Here's the drawing with two shaded views (mm, measured from the low corner). I have some questions. Round coordinates to 2 decimals unless told otherwise and drop trailing zeros. Loops run counter-clockwise (first coordinate to the right, second up) from the corner with the lowest first, then second, coordinate; pieces in that order, holes last. Notation, with made-up numbers: (40, -11.75) -> (83, -11.75) arc R35 cw to (83, 26.25) -> close; hole circle Ø5 at (39.25, 76). An arc over 180 degrees is marked (long way). Use a Markdown table: item, result.
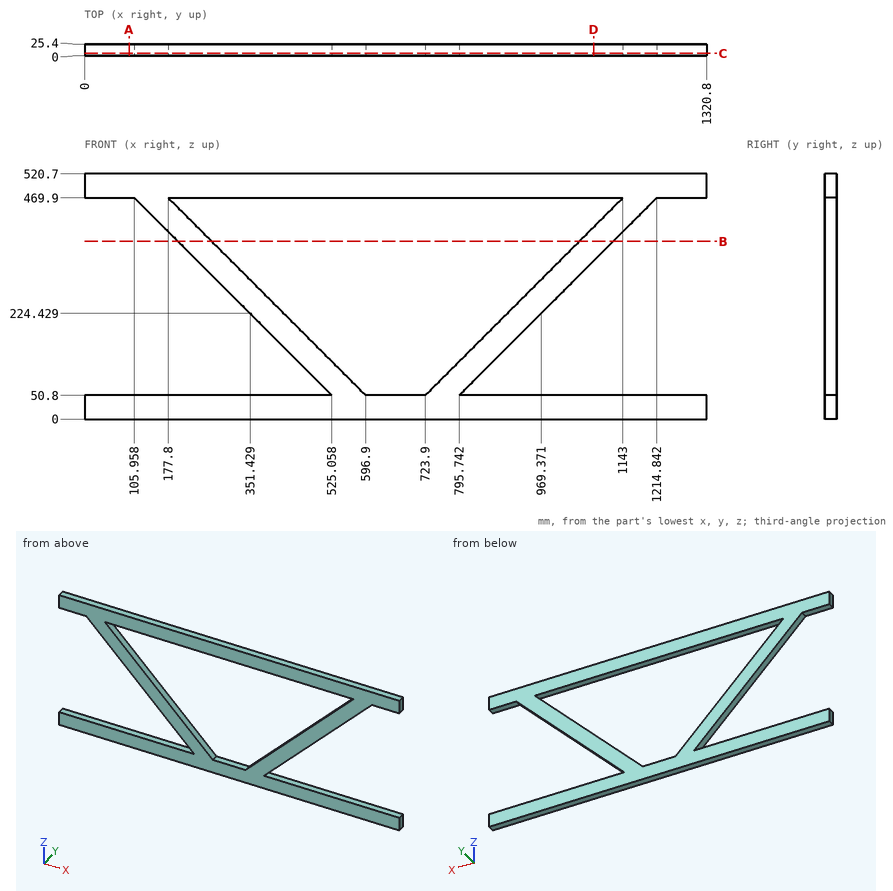
1. I want a section at B-B (z = 377.5). Please give me the cut outline in (x, y).
Answer sheet:
| item | result |
|---|---|
| outline | (198.36, 0) -> (270.2, 0) -> (270.2, 25.4) -> (198.36, 25.4) -> close; (1050.6, 0) -> (1122.44, 0) -> (1122.44, 25.4) -> (1050.6, 25.4) -> close |
2. I want a section at A-A (x = 94.5). Please give me the cut outline in (y, z), plus the area to 3 significant figures.
Answer sheet:
| item | result |
|---|---|
| outline | (0, 0) -> (25.4, 0) -> (25.4, 50.8) -> (0, 50.8) -> close; (0, 469.9) -> (25.4, 469.9) -> (25.4, 520.7) -> (0, 520.7) -> close |
| area | 2,580 mm² |
3. I want a section at D-D (x = 1081). Please give me the cut outline in (y, z), plus the area to 3 significant figures.
Answer sheet:
| item | result |
|---|---|
| outline | (0, 0) -> (25.4, 0) -> (25.4, 50.8) -> (0, 50.8) -> close; (0, 336.06) -> (25.4, 336.06) -> (25.4, 407.9) -> (0, 407.9) -> close; (0, 469.9) -> (25.4, 469.9) -> (25.4, 520.7) -> (0, 520.7) -> close |
| area | 4,410 mm² |
4. I need wall thicknesses on line 1 (Z direction, x = 486, y = 9); line 2 (Z direction, x = 1037, y = 14.75); line 3 (Z direction, x = 636, y = 6.75). Which ranges of each line are inside material? Lowest first, please.
Answer sheet:
| item | result |
|---|---|
| line 1 | z = 0 to 50.8, 89.86 to 161.7, 469.9 to 520.7 |
| line 2 | z = 0 to 50.8, 292.06 to 363.9, 469.9 to 520.7 |
| line 3 | z = 0 to 50.8, 469.9 to 520.7 |
5. Will these pins go through, and if not, where does the flat tip stop? pin 1 Ø5 at (y, z) = (17.5, 416.5) entering from +X; pin 2 Ø4 at (y, z) = (3.5, 386.5) entering from +X; pin 3 Ø10 at (y, z) = (4.5, 322) entering from +X.
Answer sheet:
| item | result |
|---|---|
| pin 1 | stops at x = 1163.94 |
| pin 2 | stops at x = 1133.44 |
| pin 3 | stops at x = 1071.94 |
6. I want a section at C-C (y = 5.5). Please give me the cut outline in (x, z).
Answer sheet:
| item | result |
|---|---|
| outline | (0, 0) -> (1320.8, 0) -> (1320.8, 50.8) -> (795.74, 50.8) -> (1214.84, 469.9) -> (1320.8, 469.9) -> (1320.8, 520.7) -> (0, 520.7) -> (0, 469.9) -> (105.96, 469.9) -> (525.06, 50.8) -> (0, 50.8) -> close; hole (177.8, 469.9) -> (596.9, 50.8) -> (723.9, 50.8) -> (1143, 469.9) -> close |
